The drawing under review shows one solid part. Ordinate dimensions are in mm from its lowest x, y, z. Give positions to 0.01 mm unless a question says otherwise; leave off trailing zeros. Write each loop counter-clockwise with the first axis right and the second up, starting at its lowest first coordinate (ties: lowest second). Pieces come first, ordered by that corner, then holes. Notation, with made-up numbers: (12.25, -7.5) -> (70.25, -7.5) arc R22 ccw to (70.25, 21.5) -> close; hole circle Ø5 at (16.5, 60). An arc over 180 degrees is marked (long way). Answer as a JSON object with one key per item and string values.
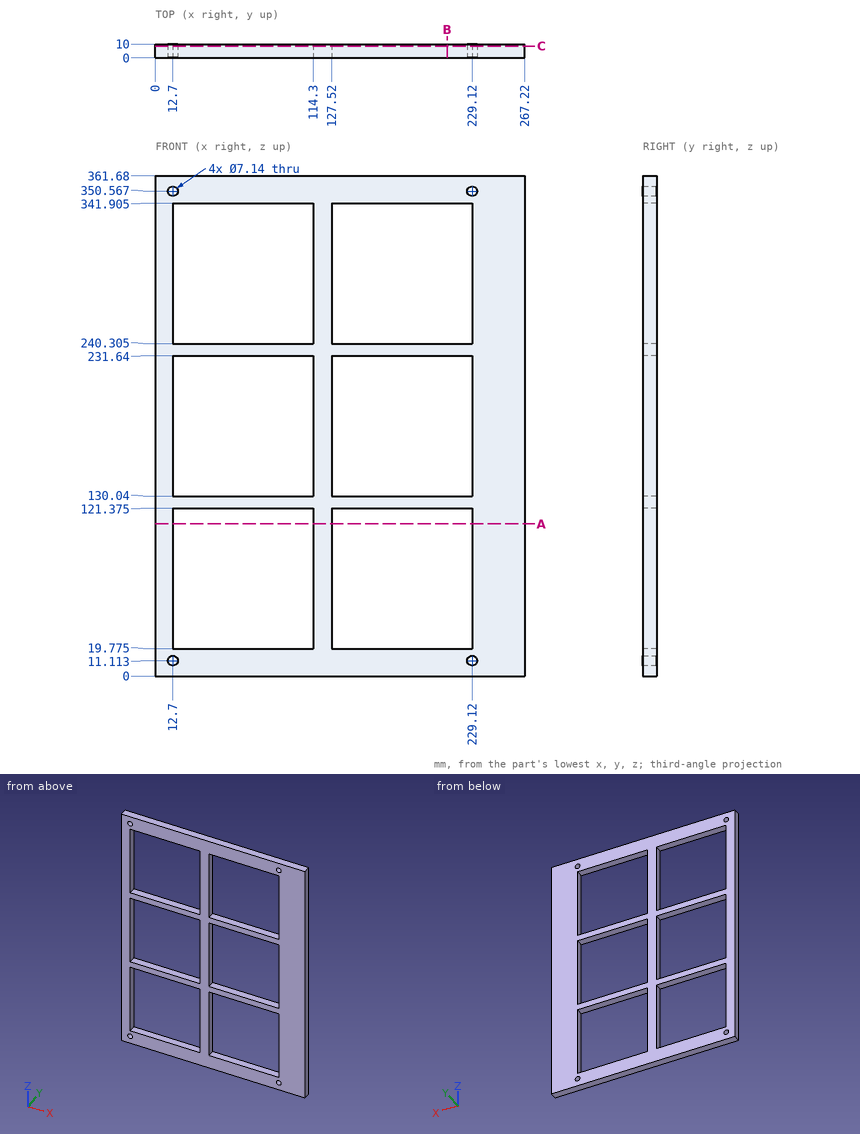
(1) We need section A-A, the plane z = 110. State the section outline as (x, y) points, then the cut area to 3 significant figures.
Here are the results:
{"outline": "(0, 0) -> (12.7, 0) -> (12.7, 10) -> (0, 10) -> close; (114.3, 0) -> (127.52, 0) -> (127.52, 10) -> (114.3, 10) -> close; (229.12, 0) -> (267.22, 0) -> (267.22, 10) -> (229.12, 10) -> close", "area": "640 mm²"}
(2) Clearance check with a flat-ended pin moving along its axis: pin 1 (4.5 mm diameter, centred on x = 229.12, z = 350.57, fed in from +Y). State where the tip first meets the part, or that it passes through.
Here are the results:
{"pin 1": "passes through"}
(3) We need section C-C, the plane y = 8.5. Give the number of separate pieces and of enclosed holes in the cut face.
Here are the results:
{"separate pieces": "1", "enclosed holes": "10"}
(4) For line 1 along Z through (x, y) = (133.5, 1.75) (1 decimal); line 2 along X through (y, z) = (4.75, 48), list the stretches that pass through material, from the lowest coordinate up.
Here are the results:
{"line 1": "z = 0 to 19.8, 121.4 to 130, 231.6 to 240.3, 341.9 to 361.7", "line 2": "x = 0 to 12.7, 114.3 to 127.52, 229.12 to 267.22"}
(5) We need section B-B, the plane x = 211. State the section outline as (y, z) points (1 decimal).
Here are the results:
{"outline": "(0, 0) -> (10, 0) -> (10, 19.8) -> (0, 19.8) -> close; (0, 121.4) -> (10, 121.4) -> (10, 130) -> (0, 130) -> close; (0, 231.6) -> (10, 231.6) -> (10, 240.3) -> (0, 240.3) -> close; (0, 341.9) -> (10, 341.9) -> (10, 361.7) -> (0, 361.7) -> close"}
